Could you check a few things on this model? Use its own coordinates, in mm. A direction names the side the tool comes from. Round coordinates to 2 decimals unless told otherwise and drop trailing zeros. Order: outer loops, then holes, each group sorted by start corner. A loop starts at its lowest first (then second) coordinate and runs counter-clockwise, first axis right, second up. Notation, with made-up numbers: (-5.5, 83) -> (30.5, 83) arc R12 ccw to (30.5, 88) -> close; hole circle Ø10 at (-14.5, 88). An arc over 180 degrees is marked (long way). One line per question, with ' | ' between items.
```python
from build123d import *

# Parameters (mm, degrees)
SKETCH_1_R               = 7
SKETCH_1_R_2             = 2.4
EXTRUDE_1_DEPTH          = 16.5
SKETCH_2_W               = 5.625
SKETCH_2_H               = 14.5
SKETCH_2_W_2             = 1.375
SKETCH_2_H_2             = 1
EXTRUDE_2_DEPTH          = 42.5
EXTRUDE_START            = -6.25
SKETCH_3_W               = 1.375
SKETCH_3_H               = 1
EXTRUDE_3_DEPTH          = 5
SKETCH_5_W               = 5.125
SKETCH_5_H               = 8
SKETCH_5_W_2             = 3.25
SKETCH_5_H_2             = 14.5
CUT_EXTRUDE_1_DEPTH      = 100.173616703
CUT_EXTRUDE_1_DEPTH_BACK = 100.173616703
CUT_EXTRUDE_2_DEPTH      = 86.750911074
CUT_EXTRUDE_2_DEPTH_BACK = 86.750911074
SKETCH_7_R               = 1.25
FILLET_1_R               = 0.25
CUT_EXTRUDE_3_DEPTH      = 100.072557411
CUT_EXTRUDE_3_DEPTH_BACK = 100.072557411
SKETCH_8_W               = 15.66616453
SKETCH_8_H               = 7.5


with BuildPart() as part:
    # Sketch 1 → Extrude 1 (new body)
    # profile 1 of 2: a face of its own
    with BuildSketch(Plane(origin=(0, -50.5, 0), x_dir=(1, 0, 0), z_dir=(0, 1, 0))):
        with Locations((58.375, 17.125)):
            Circle(SKETCH_1_R)
        with Locations(Location((58.375, 17.125, 0), (0, 0, 270))):
            Circle(SKETCH_1_R_2, mode=Mode.SUBTRACT)
    # profile 2 of 2: a face of its own
    with BuildSketch(Plane(origin=(0, -50.5, 0), x_dir=(1, 0, 0), z_dir=(0, 1, 0))):
        with BuildLine():
            Line((65.375, 10.125), (65.375, 17.125))
            ThreePointArc((65.375, 17.125), (63.324747468, 12.175252532), (58.375, 10.125))
            Line((58.375, 10.125), (65.375, 10.125))
        make_face()
    extrude(amount=EXTRUDE_1_DEPTH)

    # Sketch 2 → Extrude 2 (add)
    with BuildSketch(Plane.XY.offset(-10.125)):
        with BuildLine():
            Line((57.25, -49.5), (58.375, -49.5))
            Line((58.375, -49.5), (58.375, -35))
            Line((58.375, -35), (57.25, -35))
            ThreePointArc((57.25, -35), (50, -42.25), (57.25, -49.5))
        make_face()
        with Locations((61.1875, -42.25)):
            Rectangle(SKETCH_2_W, SKETCH_2_H)
        with Locations((64.6875, -34.5)):
            Rectangle(SKETCH_2_W_2, SKETCH_2_H_2)
        with Locations((64.6875, -42.25)):
            Rectangle(SKETCH_2_W_2, SKETCH_2_H)
        with Locations((64.6875, -50)):
            Rectangle(SKETCH_2_W_2, SKETCH_2_H_2)
    extrude(amount=EXTRUDE_2_DEPTH)

    # Sketch 3 → Extrude 3 (add)
    with BuildSketch(Plane.XY.offset(32.375).offset(EXTRUDE_START)):
        with BuildLine():
            Line((64, -49.5), (57.25, -49.5))
            ThreePointArc((57.25, -49.5), (50, -42.25), (57.25, -35))
            Line((57.25, -35), (64, -35))
            Line((64, -35), (64, -34))
            Line((64, -34), (57.25, -34))
            ThreePointArc((57.25, -34), (49, -42.25), (57.25, -50.5))
            Line((57.25, -50.5), (64, -50.5))
            Line((64, -50.5), (64, -49.5))
        make_face()
        with Locations((64.6875, -34.5)):
            Rectangle(SKETCH_3_W, SKETCH_3_H)
        with Locations((64.6875, -50)):
            Rectangle(SKETCH_3_W, SKETCH_3_H)
    extrude(amount=EXTRUDE_3_DEPTH)

    # Sketch 5 → Revolve 1 (revolve)
    with BuildSketch(Plane(origin=(0, -42.25, 0), x_dir=(1, 0, 0), z_dir=(0, 1, 0)), mode=Mode.PRIVATE) as revolve_1_sk:
        with Locations((59.8125, -36.375)):
            Rectangle(SKETCH_5_W, SKETCH_5_H)
        with Locations((58.875, -47.625)):
            Rectangle(SKETCH_5_W_2, SKETCH_5_H_2)
    revolve(revolve_1_sk.sketch.rotate(Axis((57.25, -42.25, 32.375), (0, 0, 1)), 180), axis=Axis((57.25, -42.25, 32.375), (0, 0, 1)))

    # Sketch 6 → Cut-Extrude 1 (cut, two sides: drawn at the far end of the back side and taken through both)
    with BuildSketch(Plane(origin=(0, 0, 0), x_dir=(0, 0, -1), z_dir=(1, 0, 0)).offset(-CUT_EXTRUDE_1_DEPTH_BACK)):
        Polygon((-48.25, -42.25), (-47, -39), (-54.875, -39), (-54.875, -42.25), (-53, -42.25), align=None)
        Polygon((-54.875, -45.5), (-53, -42.25), (-54.875, -42.25), align=None)
    extrude(amount=CUT_EXTRUDE_1_DEPTH + CUT_EXTRUDE_1_DEPTH_BACK, mode=Mode.SUBTRACT)

    # Sketch 7 → Cut-Extrude 2 (cut, two sides: drawn at the far end of the back side and taken through both)
    with BuildSketch(Plane(origin=(0, -42.25, 0), x_dir=(1, 0, 0), z_dir=(0, 1, 0)).offset(-CUT_EXTRUDE_2_DEPTH_BACK)):
        with Locations(Location((57.25, -50.75, 0), (0, 0, 270))):
            Circle(SKETCH_7_R)
    extrude(amount=CUT_EXTRUDE_2_DEPTH + CUT_EXTRUDE_2_DEPTH_BACK, mode=Mode.SUBTRACT)

    # Fillet 1
    fillet_1_edges = [part.edges().sort_by_distance(p)[0] for p in [
        (54.912685391, -39.99180151, 47.381462119),
        (60.5, -42.25, 50.625),
        (54.871476574, -44.464751975, 54.277741524),
        (54, -42.25, 50.625),
    ]]
    fillet(fillet_1_edges, radius=FILLET_1_R)

    # Sketch 8 → Cut-Extrude 3 (cut, two sides: drawn at the far end of the back side and taken through both)
    with BuildSketch(Plane(origin=(0, 0, 0), x_dir=(0, 0, -1), z_dir=(1, 0, 0)).offset(-CUT_EXTRUDE_3_DEPTH_BACK)):
        with Locations((17.958082265, -42.25)):
            Rectangle(SKETCH_8_W, SKETCH_8_H)
    extrude(amount=CUT_EXTRUDE_3_DEPTH + CUT_EXTRUDE_3_DEPTH_BACK, mode=Mode.SUBTRACT)


solid = part.part
```
1. I need wall thicknesses on probe 1 along Z at (x, y) = (57.25, -44.45) (3 decimals); probe 2 along Y at (x, z) = (56.75, -19); probe 3 along Z at (x, y) = (53.25, -47.25) (3 decimals). Which ranges of each line are inside material? Lowest first, please.
From the geometry:
probe 1: z = -10.125 to 49.5, 52 to 54.269 | probe 2: y = -50.5 to -46, -38.5 to -34 | probe 3: z = -21.893 to -12.357, -10.125 to 32.375
2. On a 3-axis mill with a long thin cutter (end or side, diameter ignored), from which of +Z, -Z, +X, -X, +Y, -Y can I reach the whole of each face in a straight line? I mean faces 4 (the face through (61, -35, 32)), 5 (the face through (61, -49.5, 32)), 6 (the face through (61, -49.5, 8)), 7 (the face through (49, -42.1, 28.6)). Say none if no direction works.
From the geometry:
face 4: +Z, -X, +Y | face 5: +Z, -X, -Y | face 6: -X, -Y | face 7: +Z, -X
3. I'm going to push flat-ended pins straight in: pin 1 (8 mm diameter, centred on x = 53, y = -37.5, fed in from -Z); pin 2 (1.1 mm diameter, centred on x = 60, y = -50, fed in from +Z) (3 decimals); pin 3 (3 mm diameter, centred on x = 56.5, y = -40.5, fed in from +Z); pin 4 (4 mm diameter, centred on x = 58.375, z = -17.125, fed in from +Y). Where does each tip first touch, or does it pass through?
From the geometry:
pin 1: stops at z = -23.99 | pin 2: stops at z = 32.375 | pin 3: stops at z = 48.15 | pin 4: passes through
4. If we mould it in two halves opening along Z, with no side actions, what happens to faces 1 (the face through (61, -46, 32.375)), 2 (the face through (49.8, -41.6, 26.125)), 3 (the face through (61, -46, -17))? For each: pulls with the +Z half, pulls with the -Z half, needs draft (parallel to the pull), parting line crosses it, or undercut.
From the geometry:
face 1: pulls with the +Z half | face 2: undercut | face 3: needs draft
5. I want a section at A-A on z = 50.75. List the corners of the cut face in (x, y) for me.
From the geometry:
outline: (54.01, -42.52) arc R3.25 ccw to (56, -45.25) -> (56, -42.25) -> (54.26, -42.25) arc R0.25 ccw to start; (58.5, -45.25) arc R3.25 ccw to (60.49, -42.52) arc R0.25 ccw to (60.24, -42.25) -> (58.5, -42.25) -> close
6. I want a section at C-C on z = 34. List the corners of the cut face in (x, y) for me (3 decimals).
From the geometry:
outline: circle Ø10.25 at (57.25, -42.25)
7. I want a section at B-B on z = 23. List the corners of the cut face in (x, y) for me (3 decimals), and give its area (3 significant figures).
From the geometry:
outline: (57.25, -49.5) -> (64, -49.5) -> (64, -50.5) -> (65.375, -50.5) -> (65.375, -34) -> (64, -34) -> (64, -35) -> (57.25, -35) arc R7.25 ccw to start | area: 203 mm²
